Could you check a few things on this model? Use its own coordinates, in mm. A direction names the side the tool comes from. Give positions to 0.01 mm unless a question says otherwise; leave off trailing zeros. Write each loop counter-clockwise with the first axis right and the second up, starting at its lowest first coordinate (ties: lowest second). Pieces come first, ordered by that corner, then holes. Notation, with made-up numbers: M -28,14 L 13,14 A20 cw 13,31 Z; hole C -9.5,32.5 d7. An arc over 180 degrees is marked long. Use one line per item in the form item = value.
from build123d import *

# Parameters (mm, degrees)
F1_DEPTH = 25


with BuildPart() as f1:
    # F0 (on Top) → F1 (new body)
    with BuildSketch(Plane.XY):
        with BuildLine():
            Line((-44.3664826453, 30), (-44.3664826453, 0))
            Line((-44.3664826453, 0), (-44.3664826453, -30))
            ThreePointArc((-44.3664826453, -30), (-41.4375504571, -37.0710678119), (-34.3664826453, -40))
            Line((-34.3664826453, -40), (95.6335173547, -40))
            ThreePointArc((95.6335173547, -40), (102.7045851666, -37.0710678119), (105.6335173547, -30))
            Line((105.6335173547, -30), (105.6335173547, 30))
            ThreePointArc((105.6335173547, 30), (102.7045851666, 37.0710678119), (95.6335173547, 40))
            Line((95.6335173547, 40), (-34.3664826453, 40))
            ThreePointArc((-34.3664826453, 40), (-41.4375504571, 37.0710678119), (-44.3664826453, 30))
        make_face()
        with BuildLine():
            ThreePointArc((-17.2011217286, 10.2039899685), (-16.8063733111, 10.8418548288), (-16.3879826165, 11.4644679668))
            Line((-16.3879826165, 11.4644679668), (-7.7386307522, 6.3335293543))
            ThreePointArc((-7.7386307522, 6.3335293543), (-6.8634313714, 7.2727786856), (-5.8751114363, 8.0921607505))
            Line((-5.8751114363, 8.0921607505), (-11.1341671305, 16.6141602951))
            ThreePointArc((-11.1341671305, 16.6141602951), (-10.503304654, 17.0200056212), (-9.8576667089, 17.4019081441))
            ThreePointArc((-9.8576667089, 17.4019081441), (-9.1981615432, 17.7593306244), (-8.5257169121, 18.0917702598))
            Line((-8.5257169121, 18.0917702598), (-3.5689222756, 9.341455657))
            ThreePointArc((-3.5689222756, 9.341455657), (-2.5485740405, 9.6697864692), (-1.4989449415, 9.8870199789))
            Line((-1.4989449415, 9.8870199789), (-1.4989449415, 19.94375))
            ThreePointArc((-1.4989449415, 19.94375), (-0.75, 19.9859325527), (0, 20))
            ThreePointArc((0, 20), (0.75, 19.9859325527), (1.4989449415, 19.94375))
            Line((1.4989449415, 19.94375), (1.4989449415, 9.8870199789))
            ThreePointArc((1.4989449415, 9.8870199789), (2.588190451, 9.6592582629), (3.6453855913, 9.3118829401))
            Line((3.6453855913, 9.3118829401), (8.6737506018, 18.0212666175))
            ThreePointArc((8.6737506018, 18.0212666175), (9.3434472235, 17.6833253089), (10, 17.3205080757))
            ThreePointArc((10, 17.3205080757), (10.6424853292, 16.9333253089), (11.2699993982, 16.522321676))
            Line((11.2699993982, 16.522321676), (6.2416343876, 7.8129379987))
            ThreePointArc((6.2416343876, 7.8129379987), (7.0710678119, 7.0710678119), (7.8129379987, 6.2416343876))
            Line((7.8129379987, 6.2416343876), (16.522321676, 11.2699993982))
            ThreePointArc((16.522321676, 11.2699993982), (16.9333253089, 10.6424853292), (17.3205080757, 10))
            ThreePointArc((17.3205080757, 10), (17.6833253089, 9.3434472235), (18.0212666175, 8.6737506018))
            Line((18.0212666175, 8.6737506018), (9.3118829401, 3.6453855913))
            ThreePointArc((9.3118829401, 3.6453855913), (9.6592582629, 2.588190451), (9.8870199789, 1.4989449415))
            Line((9.8870199789, 1.4989449415), (19.94375, 1.4989449415))
            ThreePointArc((19.94375, 1.4989449415), (19.9859325527, 0.75), (20, 0))
            ThreePointArc((20, 0), (19.9859325527, -0.75), (19.94375, -1.4989449415))
            Line((19.94375, -1.4989449415), (9.8870199789, -1.4989449415))
            ThreePointArc((9.8870199789, -1.4989449415), (9.6592582629, -2.588190451), (9.3118829401, -3.6453855913))
            Line((9.3118829401, -3.6453855913), (18.0212666175, -8.6737506018))
            ThreePointArc((18.0212666175, -8.6737506018), (17.6833253089, -9.3434472235), (17.3205080757, -10))
            Line((17.3205080757, -10), (16.522321676, -11.3824993982))
            Line((16.522321676, -11.3824993982), (16.4670589045, -11.3505934222))
            Line((16.4670589045, -11.3505934222), (7.7510062765, -6.3183780911))
            ThreePointArc((7.7510062765, -6.3183780911), (7.0361157976, -7.1058479073), (6.2416343876, -7.8129379987))
            Line((6.2416343876, -7.8129379987), (11.2699993982, -16.522321676))
            ThreePointArc((11.2699993982, -16.522321676), (10.6424853292, -16.9333253089), (10, -17.3205080757))
            ThreePointArc((10, -17.3205080757), (9.3434472235, -17.6833253089), (8.6737506018, -18.0212666175))
            Line((8.6737506018, -18.0212666175), (3.6453855913, -9.3118829401))
            ThreePointArc((3.6453855913, -9.3118829401), (2.588190451, -9.6592582629), (1.4989449415, -9.8870199789))
            Line((1.4989449415, -9.8870199789), (1.4989449415, -19.94375))
            ThreePointArc((1.4989449415, -19.94375), (0.75, -19.9859325527), (0, -20))
            ThreePointArc((0, -20), (-0.75, -19.9859325527), (-1.4989449415, -19.94375))
            Line((-1.4989449415, -19.94375), (-1.4989449415, -9.8870199789))
            ThreePointArc((-1.4989449415, -9.8870199789), (-2.5593257291, -9.6669463541), (-3.5896897256, -9.3334949335))
            Line((-3.5896897256, -9.3334949335), (-8.5659336261, -18.0727635162))
            ThreePointArc((-8.5659336261, -18.0727635162), (-9.237637217, -17.7388291228), (-9.8963458103, -17.3799407249))
            ThreePointArc((-9.8963458103, -17.3799407249), (-10.5411327714, -16.996603187), (-11.1710910494, -16.5893557671))
            Line((-11.1710910494, -16.5893557671), (-6.1948471489, -7.8500871844))
            ThreePointArc((-6.1948471489, -7.8500871844), (-7.0809164405, -7.0612054468), (-7.8673251482, -6.1729405482))
            Line((-7.8673251482, -6.1729405482), (-16.6204313192, -11.1248039426))
            ThreePointArc((-16.6204313192, -11.1248039426), (-17.025921115, -10.4937128885), (-17.4074597859, -9.847859859))
            ThreePointArc((-17.4074597859, -9.847859859), (-17.7645106044, -9.1881534046), (-18.0965712912, -8.5155215637))
            Line((-18.0965712912, -8.5155215637), (-9.3434651202, -3.5636581693))
            ThreePointArc((-9.3434651202, -3.5636581693), (-9.6705040957, -2.5458496686), (-9.8870199789, -1.4989449415))
            Line((-9.8870199789, -1.4989449415), (-19.94375, -1.4989449415))
            ThreePointArc((-19.94375, -1.4989449415), (-19.9859325527, -0.75), (-20, 0))
            ThreePointArc((-20, 0), (-19.9859325527, 0.75), (-19.94375, 1.4989449415))
            Line((-19.94375, 1.4989449415), (-9.8870199789, 1.4989449415))
            ThreePointArc((-9.8870199789, 1.4989449415), (-9.6437961572, 2.645221291), (-9.2681526668, 3.755175914))
            Line((-9.2681526668, 3.755175914), (-17.917504531, 8.8861145266))
            ThreePointArc((-17.917504531, 8.8861145266), (-17.5716725587, 9.5517706991), (-17.2011217286, 10.2039899685))
        make_face(mode=Mode.SUBTRACT)
        with BuildLine():
            ThreePointArc((50.7934512707, 12.0102323271), (51.1881996883, 12.6480971873), (51.6065903829, 13.2707103254))
            Line((51.6065903829, 13.2707103254), (60.2559422472, 8.1397717128))
            ThreePointArc((60.2559422472, 8.1397717128), (61.1311416279, 9.0790210442), (62.1194615631, 9.898403109))
            Line((62.1194615631, 9.898403109), (56.8604058688, 18.4204026536))
            ThreePointArc((56.8604058688, 18.4204026536), (57.4912683454, 18.8262479798), (58.1369062904, 19.2081505027))
            ThreePointArc((58.1369062904, 19.2081505027), (58.7964114562, 19.565572983), (59.4688560873, 19.8980126184))
            Line((59.4688560873, 19.8980126184), (64.4256507238, 11.1476980155))
            ThreePointArc((64.4256507238, 11.1476980155), (65.4459989589, 11.4760288278), (66.4956280579, 11.6932623374))
            Line((66.4956280579, 11.6932623374), (66.4956280579, 21.7499923586))
            ThreePointArc((66.4956280579, 21.7499923586), (67.2445729993, 21.7921749113), (67.9945729993, 21.8062423586))
            ThreePointArc((67.9945729993, 21.8062423586), (68.7445729993, 21.7921749113), (69.4935179408, 21.7499923586))
            Line((69.4935179408, 21.7499923586), (69.4935179408, 11.6932623374))
            ThreePointArc((69.4935179408, 11.6932623374), (70.5827634504, 11.4655006215), (71.6399585906, 11.1181252987))
            Line((71.6399585906, 11.1181252987), (76.6683236012, 19.827508976))
            ThreePointArc((76.6683236012, 19.827508976), (77.3380202228, 19.4895676675), (77.9945729993, 19.1267504343))
            ThreePointArc((77.9945729993, 19.1267504343), (78.6370583285, 18.7395676675), (79.2645723975, 18.3285640346))
            Line((79.2645723975, 18.3285640346), (74.236207387, 9.6191803573))
            ThreePointArc((74.236207387, 9.6191803573), (75.0656408112, 8.8773101704), (75.807510998, 8.0478767462))
            Line((75.807510998, 8.0478767462), (84.5168946753, 13.0762417567))
            ThreePointArc((84.5168946753, 13.0762417567), (84.9278983083, 12.4487276878), (85.315081075, 11.8062423586))
            ThreePointArc((85.315081075, 11.8062423586), (85.6778983083, 11.1496895821), (86.0158396168, 10.4799929604))
            Line((86.0158396168, 10.4799929604), (77.3064559395, 5.4516279498))
            ThreePointArc((77.3064559395, 5.4516279498), (77.6538312622, 4.3944328096), (77.8815929782, 3.3051873))
            Line((77.8815929782, 3.3051873), (87.9383229993, 3.3051873))
            ThreePointArc((87.9383229993, 3.3051873), (87.980505552, 2.5562423586), (87.9945729993, 1.8062423586))
            ThreePointArc((87.9945729993, 1.8062423586), (87.980505552, 1.0562423586), (87.9383229993, 0.3072974171))
            Line((87.9383229993, 0.3072974171), (77.8815929782, 0.3072974171))
            ThreePointArc((77.8815929782, 0.3072974171), (77.6538312622, -0.7819480924), (77.3064559395, -1.8391432327))
            Line((77.3064559395, -1.8391432327), (86.0158396168, -6.8675082433))
            ThreePointArc((86.0158396168, -6.8675082433), (85.6778983083, -7.5372048649), (85.315081075, -8.1937576414))
            Line((85.315081075, -8.1937576414), (84.5168946753, -9.5762570396))
            Line((84.5168946753, -9.5762570396), (84.4616319039, -9.5443510636))
            Line((84.4616319039, -9.5443510636), (75.7455792758, -4.5121357325))
            ThreePointArc((75.7455792758, -4.5121357325), (75.030688797, -5.2996055488), (74.236207387, -6.0066956401))
            Line((74.236207387, -6.0066956401), (79.2645723975, -14.7160793174))
            ThreePointArc((79.2645723975, -14.7160793174), (78.6370583285, -15.1270829504), (77.9945729993, -15.5142657171))
            ThreePointArc((77.9945729993, -15.5142657171), (77.3380202228, -15.8770829504), (76.6683236012, -16.2150242589))
            Line((76.6683236012, -16.2150242589), (71.6399585906, -7.5056405816))
            ThreePointArc((71.6399585906, -7.5056405816), (70.5827634504, -7.8530159043), (69.4935179408, -8.0807776203))
            Line((69.4935179408, -8.0807776203), (69.4935179408, -18.1375076414))
            ThreePointArc((69.4935179408, -18.1375076414), (68.7445729993, -18.1796901941), (67.9945729993, -18.1937576414))
            ThreePointArc((67.9945729993, -18.1937576414), (67.2445729993, -18.1796901941), (66.4956280579, -18.1375076414))
            Line((66.4956280579, -18.1375076414), (66.4956280579, -8.0807776203))
            ThreePointArc((66.4956280579, -8.0807776203), (65.4352472702, -7.8607039955), (64.4048832737, -7.5272525749))
            Line((64.4048832737, -7.5272525749), (59.4286393732, -16.2665211576))
            ThreePointArc((59.4286393732, -16.2665211576), (58.7569357824, -15.9325867642), (58.098227189, -15.5736983664))
            ThreePointArc((58.098227189, -15.5736983664), (57.453440228, -15.1903608284), (56.82348195, -14.7831134085))
            Line((56.82348195, -14.7831134085), (61.7997258505, -6.0438448258))
            ThreePointArc((61.7997258505, -6.0438448258), (60.9136565588, -5.2549630882), (60.1272478511, -4.3666981897))
            Line((60.1272478511, -4.3666981897), (51.3741416801, -9.3185615841))
            ThreePointArc((51.3741416801, -9.3185615841), (50.9686518844, -8.6874705299), (50.5871132135, -8.0416175004))
            ThreePointArc((50.5871132135, -8.0416175004), (50.2300623949, -7.381911046), (49.8980017081, -6.7092792051))
            Line((49.8980017081, -6.7092792051), (58.6511078791, -1.7574158107))
            ThreePointArc((58.6511078791, -1.7574158107), (58.3240689037, -0.7396073101), (58.1075530205, 0.3072974171))
            Line((58.1075530205, 0.3072974171), (48.0508229993, 0.3072974171))
            ThreePointArc((48.0508229993, 0.3072974171), (48.0086404467, 1.0562423586), (47.9945729993, 1.8062423586))
            ThreePointArc((47.9945729993, 1.8062423586), (48.0086404467, 2.5562423586), (48.0508229993, 3.3051873))
            Line((48.0508229993, 3.3051873), (58.1075530205, 3.3051873))
            ThreePointArc((58.1075530205, 3.3051873), (58.3507768422, 4.4514636496), (58.7264203326, 5.5614182726))
            Line((58.7264203326, 5.5614182726), (50.0770684683, 10.6923568852))
            ThreePointArc((50.0770684683, 10.6923568852), (50.4229004406, 11.3580130577), (50.7934512707, 12.0102323271))
        make_face(mode=Mode.SUBTRACT)
    extrude(amount=F1_DEPTH)


solid = f1.part
1) If I drill on L1, parallel to X at y = 1, z = 1.25; L2, parallel to Y at x = 79, z = 8.25; L3, parallel to Y at x = 84.5, z = 18.5, over which ranges is the centre line in solid material (lowest first)?
Checked values:
L1 = -44.37 to -19.97, 19.97 to 48.01, 87.98 to 105.63
L2 = -40 to -14.89, -14.26 to -6.39, -2.82 to 0.31, 3.31 to 6.43, 9.89 to 17.87, 18.51 to 40
L3 = -40 to -9.57, -5.99 to 0.31, 3.31 to 9.6, 13.07 to 40
2) I want a section at B-B, the plane z = 10.5. Count the separate pieces of the cut face and the enclosed holes in it, plus the area to 3 significant figures.
Checked values:
separate_pieces = 1
enclosed_holes = 2
area = 10,600 mm2
3) I want a section at A-A, the plane x = 14. Please give me the cut outline in (y, z), plus the area to 3 significant figures.
Checked values:
outline = M -40,0 L -9.93,0 L -9.93,25 L -40,25 Z; M -6.35,0 L -1.5,0 L -1.5,25 L -6.35,25 Z; M 1.5,0 L 6.35,0 L 6.35,25 L 1.5,25 Z; M 9.81,0 L 40,0 L 40,25 L 9.81,25 Z
area = 1,750 mm2
4) For pin 1 Ø5 at (y, z) = (-30.5, 14.5) entering from +X, with a flat end and sliding along its axis, tell me the tip position at first contact or that it passes through.
Checked values:
pin_1 = 105.63
5) For faces 3 (the flat face through (81.6, -4.32, 12.32)), 4 (the cylindrical face through (-41.515, -36.993, 12.325)), which set-ups out of +Z, -Z, +X, -X, +Y, -Y let a thin tool reach every point of the face, with its end or its side?
Checked values:
face_3 = +Z, -Z
face_4 = +Z, -Z, -X, -Y
6) Thinking about a two-plate mould opening in X: for faces 1 (the flat face through (-44.366, 0, 12)), 2 (the flat face through (81.72, 8, 12.32)), which applies, released by +X, released by -X, zero draft, split by the parting line, or undercut?
Checked values:
face_1 = released by -X
face_2 = undercut
